Autodesk Inventor part; units mm, degrees
ref_plane "YZ Plane" through (0, 0, 0) normal (1, 0, 0) x (0, 1, 0)
ref_plane "XZ Plane" through (0, 0, 0) normal (0, 1, 0) x (-1, 0, 0)
ref_plane "XY Plane" through (0, 0, 0) normal (0, 0, 1) x (1, 0, 0)
sketch "Sketch1" plane through (0, 0, 0) normal (1, 0, 0) x (0, 1, 0)
  line L0 (119.9441, 0) -> (-107.8442, 0)
  line L1 (140, -37.5) -> (140, -50)
  line L2 (140, -50) -> (160, -50)
  line L3 (160, -50) -> (160, -70)
  line L4 (31.9465, -37.5) -> (140, -37.5)
  line L5 (0, -150) -> (25, -150)
  line L6 (25, -150) -> (25, -90)
  line L7 (0, 154.1092) -> (0, 150) construction
  line L8 (0, -70) -> (0, -195.8423) construction
  line L9 (0, -70) -> (0, -150)
  line L10 (25, -150) -> (25, -90)
  line L11 (160, -70) -> (46.487, -70)
  line L12 (0.0098, -70) -> (0, -70)
  arc A0 (25, -90) -> (46.487, -70) centre (-38.72, 0) ccw
  arc A1 (0, -70.0054) -> (31.9465, -37.5) centre (-38.72, 0) ccw
  point P0 (0, 0)
  point P1 (150, -50)
  point P2 (18.337, -56.0758)
  dimension "d0" = 20
  dimension "d2" = 100
  dimension "d4" = 75
  dimension "d7" = 38.72
  dimension "d8" = 300
  dimension "d9" = 25
  dimension "d10" = 60
  dimension "d11" = 160
  dimension "d12" = 140
revolve "Revolution1" add sketch "Sketch1" angle 360 about axis through (0, 119.9441, 0) along (0, -1, 0) contours L1 L2 L3 L11 A0 L6 L5 L9 A1 L4
sketch "Sketch2" plane through (0, 25, 0) normal (0, 1, 0) x (1, 0, 0)
  circle A0 centre (0, -120) radius 12.5
  arc A1 (-23.3236, -133.9943) -> (23.3236, -133.9943) centre (0, -124.9939) ccw
  line L0 (0, 213.9519) -> (0, -189.1435) construction
  circle A2 centre (0, 0) radius 70
  circle A3 centre (0, 0) radius 70
  line L1 (216.3498, 0) -> (-212.0735, 0)
  circle A4 centre (0, 120) radius 12.5
  arc A5 (23.3236, 133.9943) -> (-23.3236, 133.9943) centre (0, 124.9939) ccw
  line L2 (-23.3236, 133.9943) -> (-65.3062, 25.2012)
  line L3 (-100.3964, -65.731) -> (-103.3588, -73.4078)
  line L4 (-23.3236, -133.9943) -> (-65.3062, -25.2012)
  line L5 (-100.3964, 65.731) -> (-103.3588, 73.4078)
  line L6 (23.3236, 133.9943) -> (65.3062, 25.2012)
  line L7 (100.3964, -65.731) -> (103.3588, -73.4078)
  line L8 (23.3236, -133.9943) -> (65.3062, -25.2012)
  line L9 (100.3964, 65.731) -> (103.3588, 73.4078)
  arc A6 (30.216, -116.1335) -> (30.216, 116.1335) centre (0, 0) ccw
  arc A7 (-30.216, 116.1335) -> (-30.216, -116.1335) centre (0, 0) ccw
  circle A8 centre (0, 0) radius 150.0812
  point P0 (0, -149.9939)
  point P1 (0, -120)
  point P2 (-18.02, -147.7381)
  point P3 (18.02, -147.7381)
  point P4 (-18.02, 147.7381)
  point P5 (18.02, 147.7381)
  dimension "d16" = 25
  dimension "d17" = 50
extrude "Extrusion1" cut sketch "Sketch2" along normal blind 25 and the other way blind 25 contours A0 | A1 L8 A6 L1 A8 A7 L4 | A7 L1 A2 L4 | L8 A2 L1 A6 | L1 A7 L2 A2 | L1 A8 A6 L6 A5 L2 A7 | A2 L6 A6 L1 | A4
properties part number "Quiz1"
Read the model definition and answer for the solid it produces. Units are mm, in the model's axes. A direction names the side the tool comes from. Round coordinates to 2 decimals unless told otherwise and drop trailing zeros. Loops run counter-clockwise (first coordinate to the right, second up) from the corner with the lowest first, then second, coordinate; pieces in that order, holes last.
Q1. Determine the mould class of faces 3 (the face through (-15.02, 150.14, -47.69)), 4 (the face through (-0.42, 12.32, -149.99)), 5 (the face through (0, 0, -97)), 6 (the face through (-1.627, 12.675, -132.394)) for opening direction X: released by +X, released by -X, zero draft, split by the parting line, or undercut.
Q2. Section B-B on y = 84 is taken. Write down the section's boundary in (x, z), and give its area (3 significant figures).
Q3. Each of these flat-tipped pins is pushed along its axis until it touches: pin 1 (4 mm diameter, centred on x = 34, z = 38, fed in from -Y); pin 2 (10 mm diameter, centred on x = 46, y = 75.5, fed in from -Z); pin 3 (12 mm diameter, centred on x = 5.5, y = 71, fed in from -Z). Where does it stop, or does it pass through?
Q4. Consider probe 1 along X at (y, z) = (100, 0); probe 2 along Z at (x, y) = (0, 10); probe 3 along Y at (x, z) = (13.5, -131). Determine where each line is inside the solid, lowest interval first.
Q5. Which of the six approach directions +Z, -Z, +X, -X, +Y, -Y give full straight-line access (tool end or side, diameter ignored) to faces 1 (the face through (37, 140, -7)), 2 (the face through (48.686, 17.753, 68.271))?
Q6. Section A-A on z = 120 is taken. Write down the section's boundary in (x, y), and give its area (3 significant figures).
Q7. Section C-C on y = 13 is taken. Give the number of separate pieces and of enclosed holes in the cut face, and give its area (3 significant figures).
Output:
1. face 3: undercut
1. face 4: split by the parting line
1. face 5: zero draft
1. face 6: undercut
2. outline: circle Ø140 at (0, 0); hole circle Ø75 at (0, 0)
2. area: 11,000 mm2
3. pin 1: stops at y = 21.21
3. pin 2: stops at z = -56.74
3. pin 3: stops at z = -70
4. probe 1: x = -70 to -37.5, 37.5 to 70
4. probe 2: z = -149.99 to -132.5, -107.5 to -63.45, 63.45 to 107.5, 132.5 to 149.99
4. probe 3: y = 0 to 25
5. face 1: +Y
5. face 2: +Z, +X, +Y, -Y
6. outline: (-28.72, 0) - (-12.5, 0) - (-12.5, 25) - (-28.72, 25) - close; (12.5, 0) - (28.72, 0) - (28.72, 25) - (12.5, 25) - close
6. area: 811 mm2
7. separate pieces: 1
7. enclosed holes: 3
7. area: 14,600 mm2
